```python
from build123d import *

# Parameters (mm, degrees)
SKETCH1_W          = 180
SKETCH1_H          = 160
BASE_FLANGE1_DEPTH = 0.64
EDGE_FLANGE1_DEPTH = 180
SKETCH31_R         = 2.65
CUT_EXTRUDE1_DEPTH = 185.775539507


# Sheet-metal steps are written as plain solids
with BuildPart() as part:
    # Sketch1 → Base-Flange1 (new body)
    with BuildSketch(Plane.XY):
        with Locations((0, -10)):
            Rectangle(SKETCH1_W, SKETCH1_H)
    extrude(amount=-BASE_FLANGE1_DEPTH)

    # Edge-Flange1 section (across the edge) → Edge-Flange1 (add)
    with BuildSketch(Plane(origin=(90, -91, -0.64), x_dir=(0, 1, 0), z_dir=(-1, 0, 0))):
        with BuildLine():
            Line((-0.64, 1), (-0.64, 10.36))
            Line((-0.64, 10.36), (0, 10.36))
            Line((0, 10.36), (0, 1))
            ThreePointArc((0, 1), (0.292893219, 0.292893219), (1, 0))
            Line((1, 0), (1, -0.64))
            ThreePointArc((1, -0.64), (-0.159655121, -0.159655121), (-0.64, 1))
        make_face()
    extrude(amount=EDGE_FLANGE1_DEPTH)

    # Sketch31 → Cut-Extrude1 (cut, through all)
    with BuildSketch(Plane(origin=(0, -91, 0), x_dir=(1, 0, 0), z_dir=(0, 1, 0))):
        with Locations(Location((80, 6.5, 0), (0, 0, 270))):
            Circle(SKETCH31_R)
        with Locations(Location((-80, 6.5, 0), (0, 0, 90))):
            Circle(SKETCH31_R)
    extrude(amount=-CUT_EXTRUDE1_DEPTH, mode=Mode.SUBTRACT)


solid = part.part
```
Geometry: final body of the model. Coordinates: model frame, mm. A direction names the side the tool comes from. Coordinates: 2 decimals unless noted, no trailing zeros. Loops run counter-clockwise (first coordinate to the right, second up) from the corner with the lowest first, then second, coordinate; pieces in that order, holes last. Notation, with made-up numbers: M 41.25,-18.75 L 79.25,-18.75 A16 ccw 79.25,5.25 Z; hole C 29,29.25 d6. An arc over 180 degrees is marked long. Put each result on its own line as item: value.
(1) Access query for faces 4 (the face through (-90, -10.4, -0.2)), 5 (the face through (-1, -9, -0.64)). Directions: +Z, -Z, +X, -X, +Y, -Y. A direction counts if a zero-diameter tool reaches every point of the face in a straight line with its end or side. Return the directions, or none.
Answer sheet:
face 4: +Z, -Z, -X, +Y, -Y
face 5: -Z, +X, -X, +Y
(2) First-contact query: pin 1 (3 mm diameter, centred on x = 21.5, z = -8, fed in from +Y); pin 2 (5 mm diameter, centred on x = 50, z = -2.5, fed in from +Y); pin 3 (3 mm diameter, centred on x = -80, z = -6.5, fed in from +Y). Flat tips, straight axial feed; report the tip coordinate or a pass-through.
Answer sheet:
pin 1: stops at y = -91
pin 2: stops at y = 70
pin 3: passes through
(3) Cut plane B-B on x = -1. Return the cut outline in (y, z), then the cut area to 3 significant figures.
Answer sheet:
outline: M -91.64,-11 L -91,-11 L -91,-1.64 A1 cw -90,-0.64 L 70,-0.64 L 70,0 L -90,0 A1.64 ccw -91.64,-1.64 Z
area: 110 mm^2
(4) Cut plane C-C on y = -73.5. Return the cut outline in (x, z).
Answer sheet:
outline: M -90,-0.64 L 90,-0.64 L 90,0 L -90,0 Z
(5) Draft query along X for faces 1 (the face through (-1, -9, 0)), 2 (the face through (-77.41, -91.32, -5.93)), 3 (the face through (90, -10.4, -0.2)). Return one class per face: pulls with the +X half, pulls with the -X half, needs draft (parallel to the pull), parting line crosses it, or undercut.
Answer sheet:
face 1: needs draft
face 2: undercut
face 3: pulls with the +X half
(6) Material intervals for probe 1 along X at (y, z) = (-91.4, -6.5); probe 2 along Z at (x, y) = (-80, -91.3); probe 3 along Y at (x, z) = (-54.5, -9.5), sorted ascending.
Answer sheet:
probe 1: x = -90 to -82.65, -77.35 to 77.35, 82.65 to 90
probe 2: z = -11 to -9.15, -3.85 to -0.64
probe 3: y = -91.64 to -91
(7) Cut plane A-A on z = -6.5. Return the cut outline in (x, y).
Answer sheet:
outline: M -90,-91.64 L -82.65,-91.64 L -82.65,-91 L -90,-91 Z; M -77.35,-91.64 L 77.35,-91.64 L 77.35,-91 L -77.35,-91 Z; M 82.65,-91.64 L 90,-91.64 L 90,-91 L 82.65,-91 Z
